Check sheet for the drawn part. Datum: minimum x, y, z corner. Units: mm. Round coordinates to 2 decimals unless told otherwise and drop trailing zeros. Loops run counter-clockwise (first coordinate to the right, second up) from the corner with the lowest first, then second, coordinate; pieces in that order, holes last. Notation, with made-up numbers: (84.5, 17) - (133.5, 17) arc R7 cw to (133.5, 21) - close; hole circle Ø2 at (83, 62.5). An arc over 180 degrees is marked (long way). Use CSV: the item, a comma, the result in double quotes.
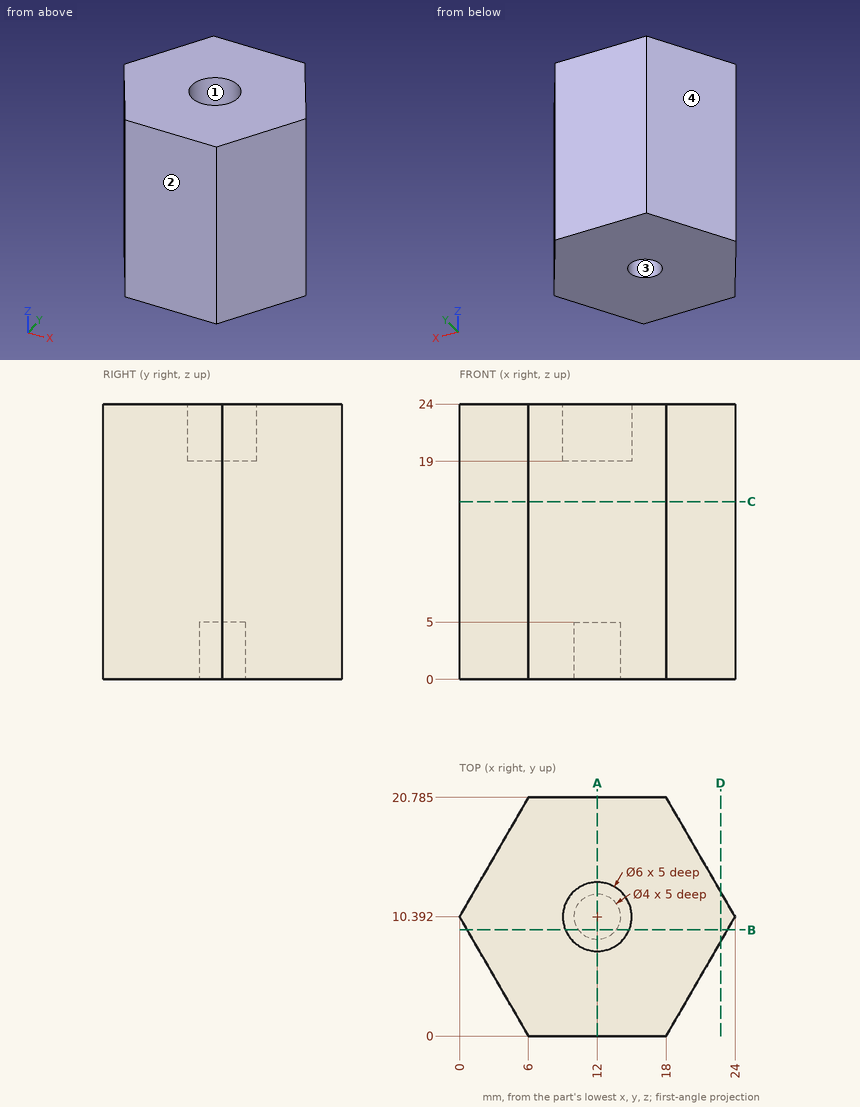
1) Cross-section at A-A, the plane x = 12. Record the cut outline in (y, z) (1 decimal), then the cut area to 3 significant figures.
Returned:
outline,"(0, 0) - (8.4, 0) - (8.4, 5) - (12.4, 5) - (12.4, 0) - (20.8, 0) - (20.8, 24) - (13.4, 24) - (13.4, 19) - (7.4, 19) - (7.4, 24) - (0, 24) - close"
area,"449 mm²"
2) Cross-section at D-D, the plane x = 22.75. Record the cut outline in (y, z), then the cut area to 3 significant figures.
Returned:
outline,"(8.23, 0) - (12.56, 0) - (12.56, 24) - (8.23, 24) - close"
area,"104 mm²"
3) Gauge pin test, flat ends, axial feed: pin 1 Ø4.5 at (x, y) = (12, 10.39) entering from +Z; pin 2 Ø1.5 at (x, z) = (5, 7.5) entering from +Y; pin 3 Ø3 at (y, z) = (2.5, 11.5) entering from +X. Record the tip position at first contact, or that the pin passes through.
Returned:
pin 1,"stops at z = 19"
pin 2,"stops at y = 20.35"
pin 3,"stops at x = 20.31"
4) Cross-section at B-B, the plane y = 9.25. Record the cut outline in (x, z).
Returned:
outline,"(0.66, 0) - (10.36, 0) - (10.36, 5) - (13.64, 5) - (13.64, 0) - (23.34, 0) - (23.34, 24) - (14.77, 24) - (14.77, 19) - (9.23, 19) - (9.23, 24) - (0.66, 24) - close"
5) Cross-section at C-C, the plane z = 15.5. Record the cut outline in (x, y) (1 decimal), then the cut area to 3 significant figures.
Returned:
outline,"(0, 10.4) - (6, 0) - (18, 0) - (24, 10.4) - (18, 20.8) - (6, 20.8) - close"
area,"374 mm²"
6) Thickness scan on probe 1 along Y at (x, z) = (12, 2.7) (1 decimal); probe 2 along Y at (x, z) = (12, 22.75) (1 decimal); probe 3 along X at (y, z) = (10.75, 19.75) (1 decimal). Record the ranges inside material, lowest first. Write a range as [from, to].
Returned:
probe 1,"y = [0, 8.4], [12.4, 20.8]"
probe 2,"y = [0, 7.4], [13.4, 20.8]"
probe 3,"x = [0.2, 9], [15, 23.8]"
7) Mould release check, pull along X, two halves, no side actions. Record for the marked faces 1, 2, 3 and 4: +X half, -X half, draft (parallel to the pull), parting line (faces both ways), or undercut.
Returned:
face 1,"undercut"
face 2,"draft"
face 3,"undercut"
face 4,"-X half"
